Source: CAD feature listing. Evaluate the final solid. Frame: model axes, mm. A direction names the side the tool comes from. Give positions to 0.01 mm unless a question says otherwise; leave off trailing zeros. Write each loop counter-clockwise with the first axis right and the second up, starting at its lowest first coordinate (ties: lowest second). Pieces come first, ordered by that corner, then holes.
Autodesk Inventor part; units mm, degrees
ref_plane "YZ Plane" through (0, 0, 0) normal (1, 0, 0) x (0, 1, 0)
ref_plane "XZ Plane" through (0, 0, 0) normal (0, 1, 0) x (-1, 0, 0)
ref_plane "XY Plane" through (0, 0, 0) normal (0, 0, 1) x (1, 0, 0)
sketch "Skizze1" plane through (0, 0, 0) normal (0, 0, 1) x (1, 0, 0)
  line L0 (-2, 0) -> (2, 0) construction
  line L1 (0, 2) -> (0, -2) construction
  line L2 (-2, 1.1547) -> (0, 2.3094)
  line L3 (0, 2.3094) -> (2, 1.1547)
  line L4 (2, 1.1547) -> (2, -1.1547)
  line L5 (2, -1.1547) -> (0, -2.3094)
  line L6 (0, -2.3094) -> (-2, -1.1547)
  line L7 (-2, -1.1547) -> (-2, 1.1547)
  point P0 (0, 0)
  point P1 (0, 0)
  point P2 (0, 0)
  dimension "d0" = 4
  dimension "d1" = 4
  dimension "d2" = 4
extrude "Extrusion1" add sketch "Skizze1" along normal mid plane 5
sketch "Skizze3" plane through (0, 0, 2.5) normal (0, 0, 1) x (1, 0, 0)
  point P0 (0, 0)
  point P1 (0, 0)
hole "Bohrung1" at (0, 0, 2.5) direction (0, 0, -1) diameter 2.013 depth 3.5 tip angle 118
sketch "Skizze4" plane through (0, 0, -2.5) normal (0, 0, -1) x (-1, 0, 0)
  circle A0 centre (0, 0) radius 1.25
  dimension "d17" = 2.5
extrude "Extrusion3" add sketch "Skizze4" along normal blind 4
thread "Gewinde2"
chamfer "Fase1" distance 0.25 angle 45 1 edges at (1.25, 0, -6.5)
properties part number "standoff (1466814)"
1. Section query C-C (x = 1.7). Return loops of the section in (y, z), plus the area to 3 significant figures.
2. Access query for faces 4 (the flat face through (1, -1, -2.5)), 5 (the cylindrical face through (0.983, 0.218, 0.726)), 6 (the flat face through (2, 0, 0)). Directions: +Z, -Z, +X, -X, +Y, -Y. A direction counts if a zero-diameter tool reaches every point of the face in a straight line with its end or side. Return the directions, or none.
3. Section query A-A (z = 1). Return loops of the section in (x, y), plus the area to 3 significant figures.
4. Line query: probe 1 along X at (y, z) = (0, -0.1); probe 2 along Z at (x, y) = (0.6, -1.35); probe 3 along X at (y, z) = (-0.8, -0.25). Output: solid intervals per line, ascending.
5. Pin query (flat end, axial travel): P1, Ø1, axis at x = -0.5, y = -2, coming from the -Z side; P2, Ø1, axis at x = -1, z = -2, coming from the -Y side. Return the tip coordinate at first contact, or that it passes through.
6. Pull-direction query (X, two-part tool) for faces 1 (the conical face through (0.05, -0.17, -1.5)), 2 (the flat face through (0, 0, -6.5)), 3 (the flat face through (0.99, 1.74, -0.04)); classes: pulls with the +X half, pulls with the -X half, needs draft (parallel to the pull), parting line crosses it, or undercut.
7. Section query B-B (z = -3). Return loops of the section in (x, y), plus the area to 3 significant figures.
The answers:
1. outline: (-1.33, -2.5) - (1.33, -2.5) - (1.33, 2.5) - (-1.33, 2.5) - close
1. area: 13.3 mm2
2. face 4: -Z
2. face 5: +Z
2. face 6: +Z, -Z, +X, +Y, -Y
3. outline: (-2, -1.15) - (0, -2.31) - (2, -1.15) - (2, 1.15) - (0, 2.31) - (-2, 1.15) - close; hole circle Ø2.01 at (0, 0)
3. area: 10.7 mm2
4. probe 1: x = -2 to -1.01, 1.01 to 2
4. probe 2: z = -2.5 to 2.5
4. probe 3: x = -2 to -0.61, 0.61 to 2
5. P1: stops at z = -2.5
5. P2: stops at y = -2.02
6. face 1: undercut
6. face 2: needs draft
6. face 3: pulls with the +X half
7. outline: circle Ø2.5 at (0, 0)
7. area: 4.91 mm2
